Input: part model. Units: mm. Frame: model coordinates. Face numbers are marked on the shaded views. A direction names the side the tool comes from. Round coordinates to 2 decimals unless told otherwise and drop trailing zeros. Write each loop counter-clockwise with the first axis right and the second up, starting at its lowest first coordinate (ties: lowest second). Pieces come first, ordered by that corner, then holes. Notation, with made-up numbers: (57, 63.5) -> (64, 63.5) arc R13 ccw to (64, 74.5) -> close; hole circle Ø1 at (0.25, 58.5). An arc over 180 degrees is marked (long way). Write item = value, one per line. Start each with the question number.
```python
from build123d import *

# Parameters (mm, degrees)
SALIENTE_EXTRUIR1_DEPTH      = 5
SALIENTE_EXTRUIR1_DEPTH_BACK = 5
CROQUIS1_R                   = 1
SALIENTE_EXTRUIR2_DEPTH      = 3
SALIENTE_EXTRUIR2_DEPTH_BACK = 3
CROQUIS2_R                   = 2


with BuildPart() as part:
    # Croquis1 → Saliente-Extruir1 (new, two sides: drawn at the far end of the back side and taken through both)
    with BuildSketch(Plane.XY.offset(-SALIENTE_EXTRUIR1_DEPTH_BACK)):
        Circle(CROQUIS1_R)
    extrude(amount=SALIENTE_EXTRUIR1_DEPTH + SALIENTE_EXTRUIR1_DEPTH_BACK)

    # Croquis2 → Saliente-Extruir2 (add, two sides: drawn at the far end of the back side and taken through both)
    with BuildSketch(Plane.XY.offset(-SALIENTE_EXTRUIR2_DEPTH_BACK)):
        Circle(CROQUIS2_R)
    extrude(amount=SALIENTE_EXTRUIR2_DEPTH + SALIENTE_EXTRUIR2_DEPTH_BACK)


solid = part.part
```
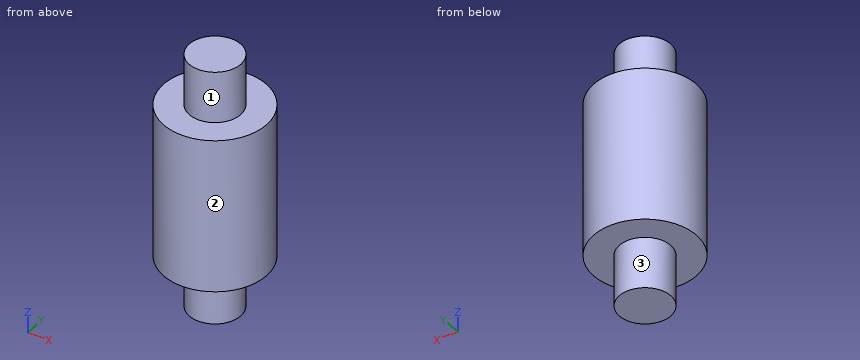
1. Pin query (flat end, axial travel): P1, Ø1, axis at x = 1, z = 1, coming from the -Y side; P2, Ø1, axis at y = 1.5, z = -1, coming from the +X side; P3, Ø1, axis at x = 1, z = 1, coming from the +Y side. Return the tip coordinate at first contact, or that it passes through.
2. Section B-B (x = 0.65). Output: boundary loops of the cut face in (y, z), then the cut area to 3 significant figures.
3. Section A-A (y = 0). Output: boundary loops of the cut face in (x, z).
4. Reachability of the marked faces 1, 2 and 3 from +Z, -Z, +X, -X, +Y, -Y: full face, straight path, thin tool, end or side. Return the list, or none.
5. Line query: line 1 along Y through (x, z) = (0.1, -0.5); line 2 along Z through (x, y) = (-1.7, 0); line 3 along X through (y, z) = (-0.5, -4). Output: solid intervals per line, ascending.
6. Section C-C (z = 3.75). Output: boundary loops of the cut face in (x, y), then the cut area to 3 significant figures.
7. Section D-D (y = -1.6). Output: boundary loops of the cut face in (x, z), then the cut area to 3 significant figures.
Check sheet entries:
q1.P1 = -1.94
q1.P2 = 1.73
q1.P3 = 1.94
q2.outline = (-1.89, -3) -> (-0.76, -3) -> (-0.76, -5) -> (0.76, -5) -> (0.76, -3) -> (1.89, -3) -> (1.89, 3) -> (0.76, 3) -> (0.76, 5) -> (-0.76, 5) -> (-0.76, 3) -> (-1.89, 3) -> close
q2.area = 28.8 mm2
q3.outline = (-2, -3) -> (-1, -3) -> (-1, -5) -> (1, -5) -> (1, -3) -> (2, -3) -> (2, 3) -> (1, 3) -> (1, 5) -> (-1, 5) -> (-1, 3) -> (-2, 3) -> close
q4.face_1 = +Z
q4.face_2 = +Z, -Z
q4.face_3 = -Z
q5.line_1 = -2 to 2
q5.line_2 = -3 to 3
q5.line_3 = -0.87 to 0.87
q6.outline = circle Ø2 at (0, 0)
q6.area = 3.14 mm2
q7.outline = (-1.2, -3) -> (1.2, -3) -> (1.2, 3) -> (-1.2, 3) -> close
q7.area = 14.4 mm2
